Verification items for the finished model (mm, model axes). A direction names the side the tool comes from. Round coordinates to 2 decimals unless told otherwise and drop trailing zeros. Write each loop counter-clockwise with the first axis right and the second up, starting at its lowest first coordinate (ties: lowest second). Pieces come first, ordered by that corner, then holes.
from build123d import *

# Parameters (mm, degrees)
PAD_DEPTH       = 3
PAD001_DEPTH    = 3
SKETCH002_W     = 209.08447
SKETCH002_H     = 4.18
PAD002_DEPTH    = 3
SKETCH003_W     = 26.3
SKETCH003_H     = 34.2
POCKET_DEPTH    = 3
SKETCH004_W     = 18
SKETCH004_H     = 25
POCKET001_DEPTH = 3
SKETCH005_W     = 14
SKETCH005_H     = 5
POCKET002_DEPTH = 6
SKETCH006_W     = 14
SKETCH006_H     = 3
POCKET003_DEPTH = 3
SKETCH007_W     = 8
SKETCH007_H     = 3
POCKET004_DEPTH = 3
SKETCH008_W     = 200
SKETCH008_H     = 4.4
PAD003_DEPTH    = 3
SKETCH009_R     = 0.8
POCKET005_DEPTH = 12


with BuildPart() as part:
    # Sketch → Pad (new body)
    with BuildSketch(Plane.XY):
        with BuildLine():
            ThreePointArc((-100, 50), (-150, 0), (-100, -50))
            Line((-100, -50), (100, -50))
            ThreePointArc((100, -50), (150, 0), (100, 50))
            Line((-100, 50), (100, 50))
        make_face()
    extrude(amount=PAD_DEPTH)

    # Sketch001 (on Face6 of Pad) → Pad001 (join)
    with BuildSketch(Plane.XY.offset(3)):
        with BuildLine():
            ThreePointArc((-100, 50), (-150, 0), (-100, -50))
            Line((-100, -50), (100, -50))
            ThreePointArc((100, -50), (150, 0), (100, 50))
            Line((-100, 50), (100, 50))
        make_face()
        with BuildLine():
            ThreePointArc((-100, 5), (-105, 0), (-100, -5))
            Line((-100, -5), (100, -5))
            ThreePointArc((100, -5), (105, 0), (100, 5))
            Line((-100, 5), (100, 5))
        make_face(mode=Mode.SUBTRACT)
    extrude(amount=PAD001_DEPTH)

    # Sketch002 (on Face9 of Pad001) → Pad002 (join)
    with BuildSketch(Plane.XY.offset(6)):
        with BuildLine():
            ThreePointArc((-100, 50), (-150, 0), (-100, -50))
            Line((-100, -50), (100, -50))
            ThreePointArc((100, -50), (150, 0), (100, 50))
            Line((-100, 50), (100, 50))
        make_face()
        Rectangle(SKETCH002_W, SKETCH002_H, mode=Mode.SUBTRACT)
    extrude(amount=PAD002_DEPTH)

    # Sketch003 (on Face13 of Pad002) → Pocket (cut)
    with BuildSketch(Plane.XY.offset(9)):
        with Locations((0, -29.9)):
            Rectangle(SKETCH003_W, SKETCH003_H)
    extrude(amount=-POCKET_DEPTH, mode=Mode.SUBTRACT)

    # Sketch004 (on Face27 of Pocket) → Pocket001 (cut)
    with BuildSketch(Plane.XY.offset(6)):
        with Locations((0, -25.3)):
            Rectangle(SKETCH004_W, SKETCH004_H)
    extrude(amount=-POCKET001_DEPTH, mode=Mode.SUBTRACT)

    # Sketch005 (on Face13 of Pocket001) → Pocket002 (cut)
    with BuildSketch(Plane.XY.offset(9)):
        with Locations((0, -10.3)):
            Rectangle(SKETCH005_W, SKETCH005_H)
    extrude(amount=-POCKET002_DEPTH, mode=Mode.SUBTRACT)

    # Sketch006 (on Face23 of Pocket002) → Pocket003 (cut)
    with BuildSketch(Plane.XZ.offset(7.8)):
        with Locations((0, 4.5)):
            Rectangle(SKETCH006_W, SKETCH006_H)
    extrude(amount=-POCKET003_DEPTH, mode=Mode.SUBTRACT)

    # Sketch007 (on Face13 of Pocket003) → Pocket004 (cut)
    with BuildSketch(Plane.XY.offset(9)):
        with Locations((0, -48.5)):
            Rectangle(SKETCH007_W, SKETCH007_H)
    extrude(amount=-POCKET004_DEPTH, mode=Mode.SUBTRACT)

    # Sketch008 (on Face15 of Pocket004) → Pad003 (join)
    with BuildSketch(Plane.XY.offset(9)):
        with BuildLine():
            ThreePointArc((-100, 50), (-150, 0), (-100, -50))
            Line((-100, -50), (100, -50))
            ThreePointArc((100, -50), (150, 0), (100, 50))
            Line((-100, 50), (100, 50))
        make_face()
        Rectangle(SKETCH008_W, SKETCH008_H, mode=Mode.SUBTRACT)
    extrude(amount=PAD003_DEPTH)

    # Sketch009 (on Face4 of Pad003) → Pocket005 (cut)
    with BuildSketch(Plane(origin=(0, 0, 0), x_dir=(1, 0, 0), z_dir=(0, 0, -1))):
        with Locations((-95, 35)):
            Circle(SKETCH009_R)
        with Locations((-95, -35)):
            Circle(SKETCH009_R)
    pocket005 = extrude(amount=-POCKET005_DEPTH, mode=Mode.SUBTRACT)

    # Mirrored: Pocket005 across Sketch009 V_Axis
    add(pocket005.mirror(Plane(origin=(0, 0, 0), x_dir=(0, 0, -1), z_dir=(1, 0, 0))), mode=Mode.SUBTRACT)


solid = part.part
Q1. Release check for a two-part mould opening along Z. For faces 3 (the flat face through (-9, -12.8, 7)), 4 (the flat face through (0, -7, 3)), 5 (the flat face through (-2, 12, 12)), 6 (the cylindrical face through (149.988, -1.099, 5.916)) record: released by +Z, released by -Z, zero draft, split by the parting line, or undercut.
Recorded:
face 3: undercut
face 4: undercut
face 5: released by +Z
face 6: zero draft
Q2. Sectioned sample at C-C (y = 19). Enter the section's corners in (x, z), plus the area to 3 significant figures.
Recorded:
outline: (-146.25, 0) - (146.25, 0) - (146.25, 12) - (-146.25, 12) - close
area: 3,510 mm2
Q3. Material ranges on line 1 along Y through (x, z) = (95, 8); line 2 along Y through (x, z) = (-95, 9.75); line 3 along Y through (x, z) = (-78, 5.5), recorded low to high.
Recorded:
line 1: y = -50 to -35.8, -34.2 to -2.09, 2.09 to 34.2, 35.8 to 50
line 2: y = -50 to -35.8, -34.2 to -2.2, 2.2 to 34.2, 35.8 to 50
line 3: y = -50 to -5, 5 to 50
Q4. Sectioned sample at D-D (y = -43). Enter the section's corners in (x, z).
Recorded:
outline: (-125.51, 0) - (125.51, 0) - (125.51, 12) - (-125.51, 12) - close; hole (-13.15, 6) - (13.15, 6) - (13.15, 9) - (-13.15, 9) - close
Q5. Depth check by flat-ended pin: P1, Ø1, axis at x = 5, y = 9.5, coming from the -Z side; P2, Ø1.5, axis at y = -30.5, z = 8, coming from the -X side; P3, Ø3, axis at y = -13.5, z = 7.5, coming from the +X side; P4, Ø1, axis at y = -27, z = 6.5, coming from the +X side. Enter the tip coordinate at first touch or a pass-through.
Recorded:
P1: stops at z = 0
P2: stops at x = -140.19
P3: stops at x = 148.54
P4: stops at x = 142.4
Q6. Tool access check on faces 1 (the flat face through (7, -10, 6)), 2 (the flat face through (-1, -50, 5)). Record the directions out of +Z, -Z, +X, -X, +Y, -Y that give a thin tool (end or side, any length) a straight path to the whole face; none if there is none.
Recorded:
face 1: none
face 2: +Z, -Z, +X, -X, -Y
Q7. Sectioned sample at B-B (x = -69.5). Enter the section's corners in (y, z), plus the area to 3 significant figures.
Recorded:
outline: (-50, 0) - (50, 0) - (50, 12) - (2.2, 12) - (2.2, 9) - (2.09, 9) - (2.09, 6) - (5, 6) - (5, 3) - (-5, 3) - (-5, 6) - (-2.09, 6) - (-2.09, 9) - (-2.2, 9) - (-2.2, 12) - (-50, 12) - close
area: 1,140 mm2
Q8. Sectioned sample at A-A (y = -15.5). Enter the section's corners in (x, z).
Recorded:
outline: (-147.54, 0) - (147.54, 0) - (147.54, 12) - (-147.54, 12) - close; hole (-13.15, 6) - (-9, 6) - (-9, 3) - (9, 3) - (9, 6) - (13.15, 6) - (13.15, 9) - (-13.15, 9) - close
